Geometry: final body of the model. Coordinates: model frame, mm. Face numbers are marked on the shaded views. A direction names the side the tool comes from. Coordinates: 2 decimals unless noted, no trailing zeros. Order: outer loops, then holes, each group sorted by start corner. A loop starts at its lowest first (then second) coordinate and runs counter-clockwise, first axis right, second up. Notation, with made-up numbers: M 25.25,35 L 74.25,35 A27 ccw 74.25,54 Z; hole C 32,27.5 d1. An arc over 180 degrees is marked long. Use CSV: the item, a comma, the result in double quotes. Start each with the question number.
1. Section query D-D on x = 5. Return the cut outline in (y, z).
2. Set-up query: the marked faces 1, 2 and 3. Return all of +Z, -Z, +X, -X, +Y, -Y with unobstructed straight access to the full face (end or side cutting, diameter ignored); none if empty.
3. Section query A-A on z = -5.2. Return the cut outline in (x, y).
4. Material intervals for line 1 (X direction, y = -3, z = -5); line 2 (Y direction, x = 12, z = 4); line 3 (Z direction, x = 5.5, y = -38.5), sorted ascending.
5. Section query C-C on y = -22.5. Return the cut outline in (x, z), and give its area (3 significant figures).
6. Section query B-B on x = 20. Return the cut outline in (y, z), and give its area (3 significant figures).
7. First-contact query: P1, Ø4, axis at x = 27.75, y = -46.42, coming from the -Z side; P2, Ø10, axis at x = 10, z = -8, coming from the +Y side; P3, Ø12, axis at x = 23, z = -14, coming from the -Y side; P4, Ø3.5, axis at x = 4.5, y = -33, coming from the +Z side. Flat tips, straight axial feed; report the tip coordinate or a pass-through.
from build123d import *

# Parameters (mm, degrees)
SKETCH_1_W          = 40
SKETCH_1_H          = 60
EXTRUDE_1_DEPTH     = 6
SKETCH_2_W          = 40
SKETCH_2_H          = 5
EXTRUDE_2_DEPTH     = 20
SKETCH_3_R          = 1.5
CUT_EXTRUDE_1_DEPTH = 20
SKETCH_5_R          = 8.5
EXTRUDE_3_DEPTH     = 5
SKETCH_7_R          = 6.5
CUT_EXTRUDE_3_DEPTH = 27
SKETCH_8_R          = 1.5
CUT_EXTRUDE_5_DEPTH = 27
SKETCH_9_W          = 20
SKETCH_9_H          = 4
CUT_EXTRUDE_6_DEPTH = 27
FILLET_1_R          = 4
FILLET_2_R          = 1


with BuildPart() as part:
    # 草图1 → 凸台-拉伸1 (new body)
    with BuildSketch(Plane.XY):
        with Locations((20, -30)):
            Rectangle(SKETCH_1_W, SKETCH_1_H)
    extrude(amount=EXTRUDE_1_DEPTH)

    # 草图2 → 凸台-拉伸2 (add)
    with BuildSketch(Plane(origin=(0, 0, 0), x_dir=(-1, 0, 0), z_dir=(0, 0, -1))):
        with Locations((-20, -2.5)):
            Rectangle(SKETCH_2_W, SKETCH_2_H)
    extrude(amount=EXTRUDE_2_DEPTH)

    # 草图3 → 切除-拉伸1 (cut)
    with BuildSketch(Plane.XY.offset(6)):
        with Locations((35.5, -33)):
            Circle(SKETCH_3_R)
        with Locations((27.75, -46.423393759)):
            Circle(SKETCH_3_R)
        with Locations((12.25, -46.423393759)):
            Circle(SKETCH_3_R)
        with Locations((4.5, -33)):
            Circle(SKETCH_3_R)
        with Locations((12.25, -19.576606241)):
            Circle(SKETCH_3_R)
        with Locations((27.75, -19.576606241)):
            Circle(SKETCH_3_R)
    extrude(amount=-CUT_EXTRUDE_1_DEPTH, mode=Mode.SUBTRACT)

    # 草图5 → 凸台-拉伸3 (add)
    with BuildSketch(Plane.XY.offset(6)):
        with Locations(Location((20, -40.3, 0), (0, 0, 214.594788024))):
            Circle(SKETCH_5_R)
    extrude(amount=EXTRUDE_3_DEPTH)

    # 草图7 → 切除-拉伸3 (cut)
    with BuildSketch(Plane.XY.offset(11)):
        with Locations((20, -40.3)):
            Circle(SKETCH_7_R)
    extrude(amount=-CUT_EXTRUDE_3_DEPTH, mode=Mode.SUBTRACT)

    # 草图8 → 切除-拉伸5 (cut)
    with BuildSketch(Plane(origin=(0, 0, 0), x_dir=(1, 0, 0), z_dir=(0, 1, 0))):
        with BuildLine():
            ThreePointArc((9.5, 14.8), (8.426322568, 16.238140837), (6.742334576, 15.617482526))
            Line((6.742334576, 15.617482526), (9.257665424, 13.982517474))
            ThreePointArc((9.257665424, 13.982517474), (9.438140837, 14.373677432), (9.5, 14.8))
        make_face()
        with BuildLine():
            Line((9.257665424, 13.982517474), (6.742334576, 15.617482526))
            ThreePointArc((6.742334576, 15.617482526), (7.182517474, 13.542334576), (9.257665424, 13.982517474))
        make_face()
        with Locations(Location((8, 5.2, 0), (0, 0, 270))):
            Circle(SKETCH_8_R)
        with Locations(Location((32, 14.8, 0), (0, 0, 270))):
            Circle(SKETCH_8_R)
        with Locations(Location((32, 5.2, 0), (0, 0, 270))):
            Circle(SKETCH_8_R)
    extrude(amount=-CUT_EXTRUDE_5_DEPTH, mode=Mode.SUBTRACT)

    # 草图9 → 切除-拉伸6 (cut)
    with BuildSketch(Plane(origin=(0, 0, 0), x_dir=(-1, 0, 0), z_dir=(0, 0, -1))):
        with Locations((-20, -55)):
            Rectangle(SKETCH_9_W, SKETCH_9_H)
    extrude(amount=-CUT_EXTRUDE_6_DEPTH, mode=Mode.SUBTRACT)

    # 圆角1
    fillet_1_edges = [part.edges().sort_by_distance(p)[0] for p in [
        (20, -5, 0),
        (20, 0, 6),
    ]]
    fillet(fillet_1_edges, radius=FILLET_1_R)

    # 圆角2
    fillet_2_edges = [part.edges().sort_by_distance(p)[0] for p in [
        (0, -34.5, 0),
        (0, -32, 6),
        (0, 0, -9),
        (0, -1.171572875, 4.828427125),
        (40, -32, 6),
        (40, 0, -9),
        (40, -1.171572875, 4.828427125),
        (0, -6.171572875, -1.171572875),
        (40, -6.171572875, -1.171572875),
        (40, -5, -12),
        (0, -5, -12),
        (20, -5, -20),
        (20, 0, -20),
        (40, -34.5, 0),
        (20, -60, 0),
        (40, -60, 3),
        (0, -60, 3),
        (20, -60, 6),
    ]]
    fillet(fillet_2_edges, radius=FILLET_2_R)


solid = part.part
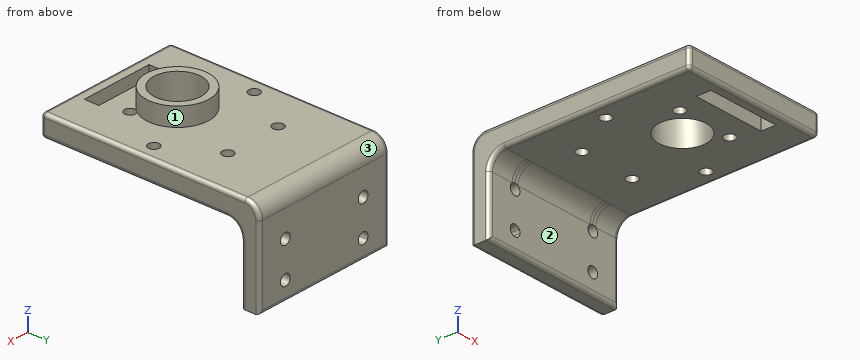
Results list:
1,outline,"M -60,1 A1 ccw -59,0 L -34.41,0 L -34.41,6 L -59,6 A1 ccw -60,5 Z; M -31.59,0 L -9,0 A4 cw -5,-4 L -5,-19 A1 ccw -4,-20 L -1,-20 A1 ccw 0,-19 L 0,2 A4 ccw -4,6 L -31.59,6 Z"
2,face 1,"+Z"
2,face 2,"-Z, +X, -X, -Y"
2,face 3,"+Z, +X, -X, +Y"
3,outline,"M 0,-4 A1 ccw 1,-5 L 6.5,-5 L 6.5,0 L 1,0 A1 ccw 0,-1 Z; M 9.5,-5 L 30.5,-5 L 30.5,0 L 9.5,0 Z; M 33.5,-5 L 39,-5 A1 ccw 40,-4 L 40,-1 A1 ccw 39,0 L 33.5,0 Z"
4,line 1,"x = 0 to 6.51, 9.49 to 30.51, 33.49 to 40"
4,line 2,"y = -60 to -57, -53 to -47.9, -44.94 to -21.06, -18.1 to -0.54"
4,line 3,"z = 0 to 6"
5,outline,"M 0,1 A1 ccw 1,0 L 39,0 A1 ccw 40,1 L 40,5 A1 ccw 39,6 L 1,6 A1 ccw 0,5 Z"
5,area,"239 mm²"
6,outline,"M -60,1 A1 ccw -59,0 L -57,0 L -57,6 L -59,6 A1 ccw -60,5 Z; M -53,0 L -46.8,0 L -46.8,11 L -48.8,11 L -48.8,6 L -53,6 Z; M -33.8,0 L -9,0 A4 cw -5,-4 L -5,-19 A1 ccw -4,-20 L -1,-20 A1 ccw 0,-19 L 0,2 A4 ccw -4,6 L -31.8,6 L -31.8,11 L -33.8,11 Z"
6,area,"377 mm²"
7,P1,"stops at z = 0"
7,P2,"stops at y = 0"
7,P3,"stops at y = -5"
7,P4,"stops at z = 6"
